For this review, take the finished solid that the model builds, in its own axes (mm). A direction names the side the tool comes from. Coordinates: 2 decimals unless noted, no trailing zeros. Write each loop counter-clockwise with the first axis right and the second up, starting at its lowest first coordinate (ties: lowest second). Pieces come first, ordered by that corner, then holes. Notation, with made-up numbers: (-39, -13) -> (1, -13) arc R17 ccw to (1, -8) -> close; hole circle Ø2 at (-4, 72). An arc over 180 degrees is marked (long way). Put each result on its own line as item: value. Start each with the question number.
Item 1: To check wall thickness, follow L1, parallel to Z at x = 9, y = 2; L2, parallel to X at y = 4.75, z = -66.5 (3 decimals); L3, parallel to Z at x = 32.5, y = 12.25. State the ranges of each line that lie inside material, in increasing order.
Item 2: Consider section B-B on z = -33.5. Give the boundary of the cut face in (x, y).
Item 3: Consider section C-C on z = -107.5. Give the boundary of the cut face in (x, y) (3 decimals).
Item 4: Consider section A-A on x = 16.75. Give the boundary of the cut face in (y, z) (3 decimals), and give its area (3 significant figures).
Item 5: Insertion check: P1, Ø1.5, axis at x = 47.5, z = -70, coming from the +Y side; P2, Ø8, axis at y = 8.5, z = -79.5, coming from the -X side; P3, Ø0.9, axis at x = 87.5, z = -80, coming from the +Y side; P4, Ø2, axis at x = 4.62, z = -44.66, coming from the +Y side. Each pin has a flat end and moves straight along its axis. Give the tip position at first contact, or say it passes through.
Item 6: Consider section D-D on x = 72. Give the boundary of the cut face in (y, z), and give its area (3 significant figures).
Item 7: For faces 1 (the flat face through (2, 10, -35)), 2 (the flat face through (90, 13, -76)), 3 (the flat face through (24.25, 1, -10)), 4 (the flat face through (0, 6, -77)), 5 (the flat face through (6.125, 8, -77)), list the 3-axis set-ups (+Z, -Z, +X, -X, +Y, -Y) from which the entire face can be reached by the end or side of a thin tool; tool diameter is ignored.
```python
from build123d import *

# Parameters (mm, degrees)
BOSS_EXTRUDE1_DEPTH = 15
SKETCH2_3_W         = 9.25
SKETCH2_3_H         = 15
SKETCH2_3_R         = 1.65
SKETCH2_3_W_2       = 15
SKETCH2_3_H_2       = 9.25
BOSS_EXTRUDE2_DEPTH = 3
SKETCH3_W           = 70
SKETCH3_H           = 96
CUT_EXTRUDE1_DEPTH  = 13
SKETCH5_W           = 9.25
SKETCH5_H           = 30.6
SKETCH5_R           = 1.3
BOSS_EXTRUDE4_DEPTH = 10
BOSS_EXTRUDE5_DEPTH = 30.6
SKETCH9_W           = 9.25
SKETCH9_H           = 35
BOSS_EXTRUDE6_DEPTH = 3
SKETCH9_4_W         = 9.25
SKETCH9_4_H         = 35
SKETCH9_4_W_2       = 3
SKETCH9_4_H_2       = 25
BOSS_EXTRUDE7_DEPTH = 13


with BuildPart() as part:
    # Sketch2 → Boss-Extrude1 (new body)
    with BuildSketch(Plane(origin=(0, 0, 0), x_dir=(1, 0, 0), z_dir=(0, 1, 0))):
        Polygon((9.25, 100), (9.25, 115), (83.25, 115), (83.25, 15), (68.25, 15), (24.25, 15), (9.25, 15), align=None)
    extrude(amount=BOSS_EXTRUDE1_DEPTH)

    # Sketch2<3> → Boss-Extrude2 (add)
    # profile 1 of 3: a face of its own
    with BuildSketch(Plane(origin=(0, 0, 0), x_dir=(1, 0, 0), z_dir=(0, 1, 0))):
        with Locations((4.625, 107.5)):
            Rectangle(SKETCH2_3_W, SKETCH2_3_H)
        with Locations(Location((4.625, 107.5, 0), (0, 0, 270))):
            Circle(SKETCH2_3_R, mode=Mode.SUBTRACT)
    # profile 2 of 3: a face of its own
    with BuildSketch(Plane(origin=(0, 0, 0), x_dir=(1, 0, 0), z_dir=(0, 1, 0))):
        with Locations((16.75, 10.375)):
            Rectangle(SKETCH2_3_W_2, SKETCH2_3_H_2)
        with Locations(Location((16.75, 10.375, 0), (0, 0, 270))):
            Circle(SKETCH2_3_R, mode=Mode.SUBTRACT)
    # profile 3 of 3: a face of its own
    with BuildSketch(Plane(origin=(0, 0, 0), x_dir=(1, 0, 0), z_dir=(0, 1, 0))):
        with Locations((75.75, 10.375)):
            Rectangle(SKETCH2_3_W_2, SKETCH2_3_H_2)
        with Locations(Location((75.75, 10.375, 0), (0, 0, 270))):
            Circle(SKETCH2_3_R, mode=Mode.SUBTRACT)
    extrude(amount=BOSS_EXTRUDE2_DEPTH)

    # Sketch3 → Cut-Extrude1 (cut)
    with BuildSketch(Plane(origin=(0, 15, 0), x_dir=(1, 0, 0), z_dir=(0, 1, 0))):
        with Locations((46.25, 65)):
            Rectangle(SKETCH3_W, SKETCH3_H)
    extrude(amount=-CUT_EXTRUDE1_DEPTH, mode=Mode.SUBTRACT)

    # Sketch5 → Boss-Extrude4 (add)
    with BuildSketch(Plane(origin=(0, 0, 0), x_dir=(1, 0, 0), z_dir=(0, 1, 0))):
        with Locations((4.625, 34.658045924)):
            Rectangle(SKETCH5_W, SKETCH5_H)
        with Locations(Location((4.625, 44.658045924, 0), (0, 0, 270))):
            Circle(SKETCH5_R, mode=Mode.SUBTRACT)
        with Locations(Location((4.625, 24.658045924, 0), (0, 0, 90))):
            Circle(SKETCH5_R, mode=Mode.SUBTRACT)
    extrude(amount=BOSS_EXTRUDE4_DEPTH)

    # Sketch6 → Boss-Extrude5 (add)
    with BuildSketch(Plane(origin=(0, 0, -49.958045924), x_dir=(-1, 0, 0), z_dir=(0, 0, -1))):
        Polygon((0, 3.177665999), (5.942499885, 10), (0, 10), align=None)
    extrude(amount=-BOSS_EXTRUDE5_DEPTH)

    # Sketch9 → Boss-Extrude6 (add)
    with BuildSketch(Plane.XZ):
        with Locations((4.625, -76.661539041)):
            Rectangle(SKETCH9_W, SKETCH9_H)
    boss_extrude6 = extrude(amount=-BOSS_EXTRUDE6_DEPTH)

    # Sketch9<4> → Boss-Extrude7 (add)
    with BuildSketch(Plane.XZ):
        with Locations((4.625, -76.661539041)):
            Rectangle(SKETCH9_4_W, SKETCH9_4_H)
        with Locations((4.625, -76.661539041)):
            Rectangle(SKETCH9_4_W_2, SKETCH9_4_H_2, mode=Mode.SUBTRACT)
    boss_extrude7 = extrude(amount=-BOSS_EXTRUDE7_DEPTH)

    # Mirror1: Boss-Extrude6, Boss-Extrude7 across plane
    add(boss_extrude6.mirror(Plane.ZY.offset(-46.25)))
    add(boss_extrude7.mirror(Plane.ZY.offset(-46.25)))


solid = part.part
```
Return value:
1. L1: -115 to -100, -94.16 to -59.16, -49.96 to -19.36
1. L2: 0 to 3.125, 6.125 to 11.25, 81.25 to 86.375, 89.375 to 92.5
1. L3: -115 to -113, -17 to -15
2. outline: (-5.94, 10) -> (0, 3.18) -> (0, 0) -> (83.25, 0) -> (83.25, 15) -> (81.25, 15) -> (81.25, 2) -> (11.25, 2) -> (11.25, 15) -> (9.25, 15) -> (9.25, 10) -> close
3. outline: (0, 0) -> (2.975, 0) -> (2.975, 3) -> (0, 3) -> close; (6.275, 0) -> (83.25, 0) -> (83.25, 15) -> (81.25, 15) -> (81.25, 2) -> (11.25, 2) -> (11.25, 15) -> (9.25, 15) -> (9.25, 3) -> (6.275, 3) -> close
4. outline: (0, -115) -> (15, -115) -> (15, -113) -> (2, -113) -> (2, -17) -> (15, -17) -> (15, -15) -> (3, -15) -> (3, -12.025) -> (0, -12.025) -> close; (0, -8.725) -> (3, -8.725) -> (3, -5.75) -> (0, -5.75) -> close
4. area: 270 mm^2
5. P1: y = 2
5. P2: x = 0
5. P3: y = 3
5. P4: through
6. outline: (0, -115) -> (15, -115) -> (15, -113) -> (2, -113) -> (2, -17) -> (15, -17) -> (15, -15) -> (3, -15) -> (3, -5.75) -> (0, -5.75) -> close
6. area: 280 mm^2
7. face 1: +Z, -X, +Y
7. face 2: +Z, -Z, +X, +Y
7. face 3: +Z, +Y, -Y
7. face 4: -Z, -X, +Y, -Y
7. face 5: +Y
